Verification items for the finished model (mm, model axes). Face numbers are marked on the shaded views. A direction names the side the tool comes from. Round coordinates to 2 decimals unless told otherwise and drop trailing zeros. Order: outer loops, then holes, each group sorted by start corner. A loop starts at its lowest first (then second) coordinate and runs counter-clockwise, first axis right, second up. Notation, with made-up numbers: (-18, 79.5) -> (23, 79.5) arc R26 cw to (23, 115.5) -> close; hole circle Ø6 at (-23, 18). An arc over 180 degrees is marked (long way). Answer in a Markdown table with one row per item. Add a question column.
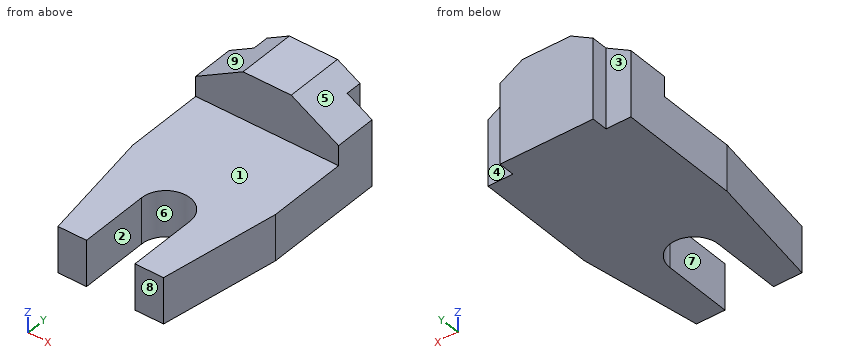
```python
from build123d import *

# Parameters (mm, degrees)
F1_DEPTH = 38.1
F2_W     = 135.403224
F2_H     = 41.598107
F3_DEPTH = 50.8
F5_DEPTH = 101.6


with BuildPart() as f1:
    # F0 (on Top) → F1 (new body)
    with BuildSketch(Plane.XY):
        with BuildLine():
            Line((16.529732, 26.053323), (16.529732, 32.657323))
            Line((16.529732, 32.657323), (-21.570268, 32.657323))
            Line((-21.570268, 32.657323), (-21.570268, 26.053323))
            Line((-21.570268, 26.053323), (-31.730268, 26.053323))
            Line((-31.730268, 26.053323), (-31.730268, -23.730677))
            Line((-31.730268, -23.730677), (-24.110268, -71.990677))
            Line((-24.110268, -71.990677), (-12.426268, -71.990677))
            Line((-12.426268, -71.990677), (-12.426268, -43.542677))
            ThreePointArc((-12.426268, -43.542677), (-2.520268, -33.636677), (7.385732, -43.542677))
            Line((7.385732, -43.542677), (7.385732, -71.990677))
            Line((7.385732, -71.990677), (19.069732, -71.990677))
            Line((19.069732, -71.990677), (26.689732, -23.730677))
            Line((26.689732, -23.730677), (26.689732, 26.053323))
            Line((26.689732, 26.053323), (16.529732, 26.053323))
        make_face()
    extrude(amount=F1_DEPTH)

    # F2 (on Right) → F3 (cut, symmetric)
    with BuildSketch(Plane.YZ):
        with Locations((-58.920289, 39.595053)):
            Rectangle(F2_W, F2_H)
    extrude(amount=F3_DEPTH, both=True, mode=Mode.SUBTRACT)

    # F4 (on Front) → F5 (cut)
    with BuildSketch(Plane.XZ):
        Polygon((26.689732, 26.924), (26.689732, 38.1), (7.332333, 38.1), align=None)
        Polygon((-31.730268, 26.924), (-12.372868, 38.1), (-31.730268, 38.1), align=None)
    extrude(amount=-F5_DEPTH, mode=Mode.SUBTRACT)


solid = f1.part
```
1) Cross-section at D-D, the plane y = -19. Record the boundary of the cut face in (x, z), and give its area (3 significant figures).
2) Tool access check on the marked faces 1, 2, 3, 4 and 5. Record the directions out of +Z, -Z, +X, -X, +Y, -Y that give a thin tool (end or side, any length) a straight path to the whole face; none if there is none.
3) Depth check by flat-ended pin: P1, Ø3, axis at x = 22.5, z = 18, coming from the +Y side; P2, Ø5.5, axis at y = 29, z = 24, coming from the -X side; P3, Ø15, axis at y = -62, z = 8, coming from the -X side. Enter the tip coordinate at first touch or a pass-through.
4) Draft check along X on the marked faces 6, 7, 8 and 9. Enter one of: +X half, -X half, draft (parallel to the pull), parting line (faces both ways), or undercut.
5) Cross-section at B-B, the plane y = -47.5. Record the boundary of the cut face in (x, z), and give its area (3 significant figures).
6) Thickness scan on L1, parallel to Z at x = -1, y = -13; L2, parallel to Y at x = -7, z = 31.5; L3, parallel to X at y = -45, z = 3. Record the ranges inside material, lowest first. Write a range as [from, to].
7) Cross-section at C-C, the plane x = 22. Record the boundary of the cut face in (y, z).
8) Cross-section at A-A, the plane z = 25.5. Record the boundary of the cut face in (x, y).
Results below:
| question | item | result |
|---|---|---|
| 1 | outline | (-31.73, 0) -> (26.69, 0) -> (26.69, 18.8) -> (-31.73, 18.8) -> close |
| 1 | area | 1,100 mm² |
| 2 | face 1 | +Z, +X, -X, -Y |
| 2 | face 2 | +Z, -Z, -Y |
| 2 | face 3 | +Z, -Z, -X, +Y |
| 2 | face 4 | +Z, -Z, +X, +Y |
| 2 | face 5 | +Z, +X, +Y, -Y |
| 3 | P1 | y = 26.05 |
| 3 | P2 | x = -21.57 |
| 3 | P3 | x = -26.87 |
| 4 | face 6 | undercut |
| 4 | face 7 | undercut |
| 4 | face 8 | draft |
| 4 | face 9 | -X half |
| 5 | outline | (-27.98, 0) -> (-12.43, 0) -> (-12.43, 18.8) -> (-27.98, 18.8) -> close; (7.39, 0) -> (22.94, 0) -> (22.94, 18.8) -> (7.39, 18.8) -> close |
| 5 | area | 585 mm² |
| 6 | L1 | [0, 18.8] |
| 6 | L2 | [8.78, 32.66] |
| 6 | L3 | [-28.37, -12.43], [7.39, 23.33] |
| 7 | outline | (-53.43, 0) -> (26.05, 0) -> (26.05, 29.63) -> (8.78, 29.63) -> (8.78, 18.8) -> (-53.43, 18.8) -> close |
| 8 | outline | (-31.73, 8.78) -> (26.69, 8.78) -> (26.69, 26.05) -> (16.53, 26.05) -> (16.53, 32.66) -> (-21.57, 32.66) -> (-21.57, 26.05) -> (-31.73, 26.05) -> close |
